For this review, take the finished solid that the model builds, in its own axes (mm). Face numbers are marked on the shaded views. A direction names the side the tool comes from. Round coordinates to 2 decimals unless told otherwise and drop trailing zeros. Order: outer loops, then holes, each group sorted by start corner. A loop starts at its lowest first (then second) coordinate and runs counter-clockwise, first axis right, second up. Notation, with made-up numbers: (25.5, -19) - (82.5, -19) arc R20 cw to (82.5, -11) - close; hole circle Ø2 at (29, 15). An arc over 180 degrees is marked (long way). Write each question's results on one line, items separated by ' | '. Start each with the question number.
(1) Take a section at B-B, the plane y = 0. Give the boundary of the cut face in (x, z).
(2) Insertion check: pin 1 Ø1.5 at (x, y) = (158, 0) entering from +Z. The pin has a flat end and moves straight along its axis. Give the tip position at first contact, or say it passes through.
(3) For L1, parallel to X at y = 2.15, z = 56.5; L2, parallel to Z at x = 175, y = -1; L3, parallel to Z at x = 192, y = 1.2, list the stretches that pass through material, from the lowest coordinate up. Write a range as from..to.
(4) Take a section at A-A, the plane z = 55. Give the boundary of the cut face in (x, y).
(5) Take a section at C-C, the plane x = 165. Give the boundary of the cut face in (y, z), plus the area to 3 significant figures.
(6) For the marked faces 1, 2 and 3, list the 3-axis set-ups (+Z, -Z, +X, -X, +Y, -Y) from which the entire face can be reached by the end or side of a thin tool; tool diameter is ignored.
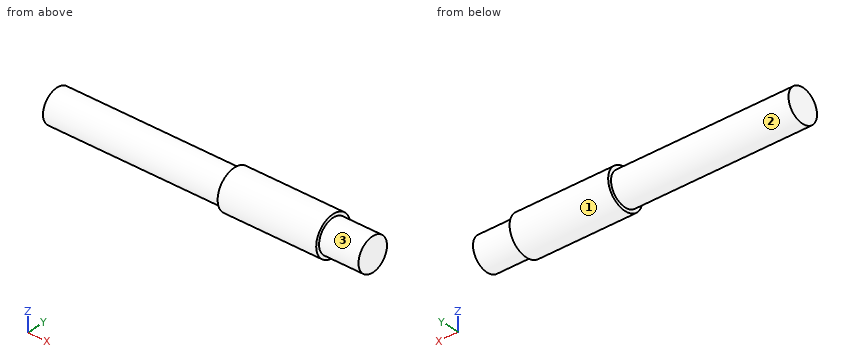
```python
from build123d import *

# Parameters (mm, degrees)
CYLINDER1492253_R     = 2.5
CYLINDER1492253_DEPTH = 48
CYLINDER1492303_R     = 3
CYLINDER1492303_DEPTH = 15


with BuildPart() as cylinder:
    # Cylinder1492253 → Cylinder1492253 (new body)
    with BuildSketch(Plane(origin=(152, 0, 55), x_dir=(0, 0, -1), z_dir=(1, 0, 0))):
        Circle(CYLINDER1492253_R)
    extrude(amount=CYLINDER1492253_DEPTH)


with BuildPart() as gearbox_shaft_steel:
    # Cylinder1492303 → Cylinder1492303 (new body)
    with BuildSketch(Plane(origin=(179, 0, 55), x_dir=(0, 0, -1), z_dir=(1, 0, 0))):
        Circle(CYLINDER1492303_R)
    extrude(amount=CYLINDER1492303_DEPTH)

    # Fusion: union Cylinder
    add(cylinder.part)


solid = gearbox_shaft_steel.part
```
Results below:
1) outline: (152, 52.5) - (179, 52.5) - (179, 52) - (194, 52) - (194, 52.5) - (200, 52.5) - (200, 57.5) - (194, 57.5) - (194, 58) - (179, 58) - (179, 57.5) - (152, 57.5) - close
2) pin 1: stops at z = 57.5
3) L1: x = 179..194 | L2: z = 52.71..57.29 | L3: z = 52.25..57.75
4) outline: (152, -2.5) - (179, -2.5) - (179, -3) - (194, -3) - (194, -2.5) - (200, -2.5) - (200, 2.5) - (194, 2.5) - (194, 3) - (179, 3) - (179, 2.5) - (152, 2.5) - close
5) outline: circle Ø5 at (0, 55) | area: 19.6 mm^2
6) face 1: +X, -X | face 2: -X | face 3: +X
